For this review, take the finished solid that the model builds, in its own axes (mm). A direction names the side the tool comes from. Give positions to 0.01 mm unless a question says otherwise; leave off trailing zeros. Order: outer loops, then holes, each group sorted by start corner. A loop starts at its lowest first (then second) coordinate and runs counter-clockwise, first axis right, second up.
from build123d import *

# Parameters (mm, degrees)
F1_DEPTH = 15
F3_DEPTH = 30
F2_R     = 2.5
F4_DEPTH = 34


with BuildPart() as f1:
    # F0 (on Top) → F1 (new body)
    with BuildSketch(Plane.XY):
        with BuildLine():
            ThreePointArc((9.032456, 4.29124), (9.755116, 2.199482), (10, 0))
            ThreePointArc((10, 0), (9.855601, -1.693258), (9.426575, -3.337616))
            Line((9.426575, -3.337616), (28.279726, -10.012847))
            ThreePointArc((28.279726, -10.012847), (29.566804, -5.079775), (30, 0))
            ThreePointArc((30, 0), (29.26777, 6.587689), (27.106824, 12.853797))
            Line((27.106824, 12.853797), (27.064093, 12.85387))
            Line((27.064093, 12.85387), (27.055619, 12.853885))
            Line((27.055619, 12.853885), (9.032456, 4.29124))
        make_face()
        with BuildLine():
            ThreePointArc((3.46339, 9.381094), (6.746347, 7.381518), (9.032456, 4.29124))
            Line((9.032456, 4.29124), (27.055619, 12.853885))
            Line((27.055619, 12.853885), (27.07179, 12.861568))
            Line((27.07179, 12.861568), (27.093042, 12.88282))
            ThreePointArc((27.093042, 12.88282), (20.136379, 22.237946), (10.13882, 28.234807))
            Line((10.13882, 28.234807), (3.46339, 9.381094))
        make_face()
        with BuildLine():
            Line((28.279726, -10.012847), (9.426575, -3.337616))
            ThreePointArc((9.426575, -3.337616), (7.472968, -6.644904), (4.416744, -8.971754))
            Line((4.416744, -8.971754), (12.999502, -27.037251))
            ThreePointArc((12.999502, -27.037251), (22.302768, -20.064559), (28.256426, -10.078412))
            Line((28.256426, -10.078412), (28.226262, -10.048145))
            Line((28.226262, -10.048145), (28.267203, -10.048145))
            ThreePointArc((28.267203, -10.048145), (28.27347, -10.030498), (28.279726, -10.012847))
        make_face()
        with BuildLine():
            ThreePointArc((-4.24614, 9.053745), (-0.424222, 9.990998), (3.46339, 9.381094))
            Line((3.46339, 9.381094), (10.13882, 28.234807))
            ThreePointArc((10.13882, 28.234807), (10.108621, 28.245633), (10.078412, 28.256426))
            Line((10.078412, 28.256426), (10.048145, 28.226262))
            Line((10.048145, 28.226262), (10.048145, 28.267203))
            ThreePointArc((10.048145, 28.267203), (-1.50418, 29.962267), (-12.828655, 27.118732))
            Line((-12.828655, 27.118732), (-4.24614, 9.053745))
        make_face()
        with BuildLine():
            Line((12.999502, -27.037251), (4.416744, -8.971754))
            ThreePointArc((4.416744, -8.971754), (0.617235, -9.980933), (-3.277666, -9.447587))
            Line((-3.277666, -9.447587), (-9.952942, -28.300865))
            ThreePointArc((-9.952942, -28.300865), (1.568494, -29.958969), (12.853797, -27.106824))
            Line((12.853797, -27.106824), (12.85387, -27.064093))
            Line((12.85387, -27.064093), (12.88282, -27.093042))
            ThreePointArc((12.88282, -27.093042), (12.941191, -27.06521), (12.999502, -27.037251))
        make_face()
        with BuildLine():
            ThreePointArc((-9.402907, 3.403723), (-7.386123, 6.741305), (-4.24614, 9.053745))
            Line((-4.24614, 9.053745), (-12.828655, 27.118732))
            ThreePointArc((-12.828655, 27.118732), (-22.239146, 20.135053), (-28.256213, 10.079009))
            Line((-28.256213, 10.079009), (-9.402907, 3.403723))
        make_face()
        with BuildLine():
            Line((27.07179, 12.861568), (27.064093, 12.85387))
            Line((27.064093, 12.85387), (27.106824, 12.853797))
            ThreePointArc((27.106824, 12.853797), (27.102098, 12.863759), (27.097368, 12.873719))
            Line((27.097368, 12.873719), (27.07179, 12.861568))
        make_face()
        with BuildLine():
            Line((27.093042, 12.88282), (27.07179, 12.861568))
            Line((27.07179, 12.861568), (27.097368, 12.873719))
            ThreePointArc((27.097368, 12.873719), (27.095206, 12.87827), (27.093042, 12.88282))
        make_face()
        with BuildLine():
            Line((-9.952942, -28.300865), (-3.277666, -9.447587))
            ThreePointArc((-3.277666, -9.447587), (-6.639802, -7.477502), (-8.993671, -4.371943))
            Line((-8.993671, -4.371943), (-27.058824, -12.954537))
            ThreePointArc((-27.058824, -12.954537), (-20.083091, -22.286083), (-10.078412, -28.256426))
            Line((-10.078412, -28.256426), (-10.048145, -28.226262))
            Line((-10.048145, -28.226262), (-10.048145, -28.267203))
            ThreePointArc((-10.048145, -28.267203), (-10.000557, -28.284074), (-9.952942, -28.300865))
        make_face()
        with BuildLine():
            ThreePointArc((28.256426, -10.078412), (28.261819, -10.06328), (28.267203, -10.048145))
            Line((28.267203, -10.048145), (28.226262, -10.048145))
            Line((28.226262, -10.048145), (28.256426, -10.078412))
        make_face()
        with BuildLine():
            ThreePointArc((-8.993671, -4.371943), (-9.986179, -0.525577), (-9.402907, 3.403723))
            Line((-9.402907, 3.403723), (-28.256213, 10.079009))
            ThreePointArc((-28.256213, 10.079009), (-28.25632, 10.07871), (-28.256426, 10.078412))
            Line((-28.256426, 10.078412), (-28.226262, 10.048145))
            Line((-28.226262, 10.048145), (-28.267203, 10.048145))
            ThreePointArc((-28.267203, 10.048145), (-29.961566, -1.518072), (-27.106824, -12.853797))
            Line((-27.106824, -12.853797), (-27.064093, -12.85387))
            Line((-27.064093, -12.85387), (-27.093042, -12.88282))
            ThreePointArc((-27.093042, -12.88282), (-27.075957, -12.91869), (-27.058824, -12.954537))
            Line((-27.058824, -12.954537), (-8.993671, -4.371943))
        make_face()
        with BuildLine():
            Line((10.048145, 28.226262), (10.078412, 28.256426))
            ThreePointArc((10.078412, 28.256426), (10.06328, 28.261819), (10.048145, 28.267203))
            Line((10.048145, 28.267203), (10.048145, 28.226262))
        make_face()
        with BuildLine():
            ThreePointArc((12.853797, -27.106824), (12.86831, -27.099937), (12.88282, -27.093042))
            Line((12.88282, -27.093042), (12.85387, -27.064093))
            Line((12.85387, -27.064093), (12.853797, -27.106824))
        make_face()
        with BuildLine():
            ThreePointArc((-10.078412, -28.256426), (-10.06328, -28.261819), (-10.048145, -28.267203))
            Line((-10.048145, -28.267203), (-10.048145, -28.226262))
            Line((-10.048145, -28.226262), (-10.078412, -28.256426))
        make_face()
        with BuildLine():
            Line((-28.226262, 10.048145), (-28.256426, 10.078412))
            ThreePointArc((-28.256426, 10.078412), (-28.261819, 10.06328), (-28.267203, 10.048145))
            Line((-28.267203, 10.048145), (-28.226262, 10.048145))
        make_face()
        with BuildLine():
            ThreePointArc((-27.106824, -12.853797), (-27.099937, -12.86831), (-27.093042, -12.88282))
            Line((-27.093042, -12.88282), (-27.064093, -12.85387))
            Line((-27.064093, -12.85387), (-27.106824, -12.853797))
        make_face()
    extrude(amount=F1_DEPTH)

    # F0 (on Top) → F3 (join)
    with BuildSketch(Plane.XY):
        with BuildLine():
            ThreePointArc((-4.24614, 9.053745), (-0.424222, 9.990998), (3.46339, 9.381094))
            Line((3.46339, 9.381094), (10.13882, 28.234807))
            ThreePointArc((10.13882, 28.234807), (10.108621, 28.245633), (10.078412, 28.256426))
            Line((10.078412, 28.256426), (10.048145, 28.226262))
            Line((10.048145, 28.226262), (10.048145, 28.267203))
            ThreePointArc((10.048145, 28.267203), (-1.50418, 29.962267), (-12.828655, 27.118732))
            Line((-12.828655, 27.118732), (-4.24614, 9.053745))
        make_face()
        with BuildLine():
            Line((12.999502, -27.037251), (4.416744, -8.971754))
            ThreePointArc((4.416744, -8.971754), (0.617235, -9.980933), (-3.277666, -9.447587))
            Line((-3.277666, -9.447587), (-9.952942, -28.300865))
            ThreePointArc((-9.952942, -28.300865), (1.568494, -29.958969), (12.853797, -27.106824))
            Line((12.853797, -27.106824), (12.85387, -27.064093))
            Line((12.85387, -27.064093), (12.88282, -27.093042))
            ThreePointArc((12.88282, -27.093042), (12.941191, -27.06521), (12.999502, -27.037251))
        make_face()
        with BuildLine():
            ThreePointArc((-8.993671, -4.371943), (-9.986179, -0.525577), (-9.402907, 3.403723))
            Line((-9.402907, 3.403723), (-28.256213, 10.079009))
            ThreePointArc((-28.256213, 10.079009), (-28.25632, 10.07871), (-28.256426, 10.078412))
            Line((-28.256426, 10.078412), (-28.226262, 10.048145))
            Line((-28.226262, 10.048145), (-28.267203, 10.048145))
            ThreePointArc((-28.267203, 10.048145), (-29.961566, -1.518072), (-27.106824, -12.853797))
            Line((-27.106824, -12.853797), (-27.064093, -12.85387))
            Line((-27.064093, -12.85387), (-27.093042, -12.88282))
            ThreePointArc((-27.093042, -12.88282), (-27.075957, -12.91869), (-27.058824, -12.954537))
            Line((-27.058824, -12.954537), (-8.993671, -4.371943))
        make_face()
        with BuildLine():
            ThreePointArc((9.032456, 4.29124), (9.755116, 2.199482), (10, 0))
            ThreePointArc((10, 0), (9.855601, -1.693258), (9.426575, -3.337616))
            Line((9.426575, -3.337616), (28.279726, -10.012847))
            ThreePointArc((28.279726, -10.012847), (29.566804, -5.079775), (30, 0))
            ThreePointArc((30, 0), (29.26777, 6.587689), (27.106824, 12.853797))
            Line((27.106824, 12.853797), (27.064093, 12.85387))
            Line((27.064093, 12.85387), (27.055619, 12.853885))
            Line((27.055619, 12.853885), (9.032456, 4.29124))
        make_face()
    extrude(amount=F3_DEPTH)

    # F2 (on Right) → F4 (cut)
    with BuildSketch(Plane.YZ):
        with Locations((0, 8.289474)):
            Circle(F2_R)
    extrude(amount=F4_DEPTH, mode=Mode.SUBTRACT)


solid = f1.part
1) To check wall thickness, follow line 1 (Z direction, x = 9.5, y = 12.5); line 2 (Y direction, x = 24.5, z = 9.5); line 3 (Y direction, x = 2, z = 5.5). State the ranges of each line that lie inside material, in increasing order.
Answer sheet:
line 1: z = 0 to 15
line 2: y = -17.31 to -2.19, 2.19 to 17.31
line 3: y = -29.93 to -9.8, 9.8 to 29.93
2) We need section C-C on x = -5. Give the boundary of the cut face in (y, z).
Answer sheet:
outline: (-29.58, 0) - (-8.66, 0) - (-8.66, 15) - (-14.31, 15) - (-14.31, 30) - (-29.58, 30) - close; (8.66, 0) - (29.58, 0) - (29.58, 30) - (10.64, 30) - (10.64, 15) - (8.66, 15) - close
3) Tool access review of faces 4 (the face through (-16, 15, 15)), 5 (the face through (22.19, -20.19, 7.4)), 6 (the face through (20, -1, 6)), 7 (the face through (1, -22, 30)), 8 (the face through (9.86, -1.67, 14.79)): name each direction out of +Z, -Z, +X, -X, +Y, -Y from which nothing blocks a thin tool from reaching the whole face with its end or side.
Answer sheet:
face 4: +Z
face 5: +Z, -Z, +X, -Y
face 6: +X
face 7: +Z, +X, -X, +Y, -Y
face 8: +Z, -Z
4) Clearance check with flat-ended pins moving along their axes: pin 1 (1.5 mm diameter, centred on y = -21, z = 16.5, fed in from +X); pin 2 (3 mm diameter, centred on y = 0, z = 8.29, fed in from +X); pin 3 (3 mm diameter, centred on x = 6, z = 6.5, fed in from +Y). State where each tip first meets the part, or that it passes through.
Answer sheet:
pin 1: stops at x = 10.49
pin 2: stops at x = -9.89
pin 3: stops at y = 29.66
5) We need section A-A on z = 25.5. Count the separate pieces of the cut face and the enclosed holes in it, then the cut area to 3 significant figures.
Answer sheet:
separate pieces: 4
enclosed holes: 0
area: 1,260 mm2
6) Draft analysis for pull direction Y (two halves, no side actions). For faces 1 (the face through (20.258, 22.127, 7.395)), 2 (the face through (-8.597, 18.213, 22.395)), 3 (the face through (-22, -1, 30)), state which applies: +Y half, -Y half, draft (parallel to the pull), parting line (faces both ways), or undercut.
Answer sheet:
face 1: +Y half
face 2: undercut
face 3: draft
7) We need section B-B on y = -1. Give the boundary of the cut face in (x, z).
Answer sheet:
outline: (-29.98, 0) - (-9.95, 0) - (-9.95, 30) - (-29.98, 30) - close; (9.95, 0) - (29.98, 0) - (29.98, 6) - (9.95, 6) - close; (9.95, 10.58) - (29.98, 10.58) - (29.98, 30) - (9.95, 30) - close
8) We need section D-D on y = -17. Give the boundary of the cut face in (x, z), then the cut area to 3 significant figures.
Answer sheet:
outline: (-24.72, 0) - (24.72, 0) - (24.72, 15) - (8.23, 15) - (8.23, 30) - (-5.95, 30) - (-5.95, 15) - (-24.72, 15) - close
area: 954 mm2
